Study the drawing (mm; zero at the part's minimum x, y, z) and answer. Coordinates: 2 decimals unless noted, no trailing zeros. Loops run counter-clockwise (first coordinate to the right, second up) from the corner with the lowest first, then second, coordinate; pieces in that order, holes last. Notation, with made-up numbers: (27.5, 41.25) - (38.5, 41.25) arc R17 cw to (38.5, 53.25) - close; hole circle Ø1 at (59, 28). An arc over 180 degrees is marked (long way). Write each question's results on one line, items separated by ' | '. Start each with the question number.
(1) Find section B-B on x = 28. Determine the outline of the cut face in (y, z).
(2) Find section C-C on z = 3.15. Determine the outline of the cut face in (x, y), then the cut area to 3 significant figures.
(3) Given pin 1 Ø1.5 at (x, z) = (66.5, 3) entering from +Y; pin 2 Ø5 at (x, y) = (95.165, 2.79) entering from +Z; pin 3 Ø2 at (y, z) = (18.5, 3.5) entering from -X, each flat-ended and moving along its own axis, determine where each tip first touches the part or whether it passes through.
(4) Consider line 1 (Y direction, x = 59.5, z = 2.3); line 2 (X direction, y = 3, z = 2.9). Determine where each line is inside the solid, lowest interval first. Write a range as from..to.
(5) Find section A-A on y = 49.5. Determine the outline of the cut face in (x, z).
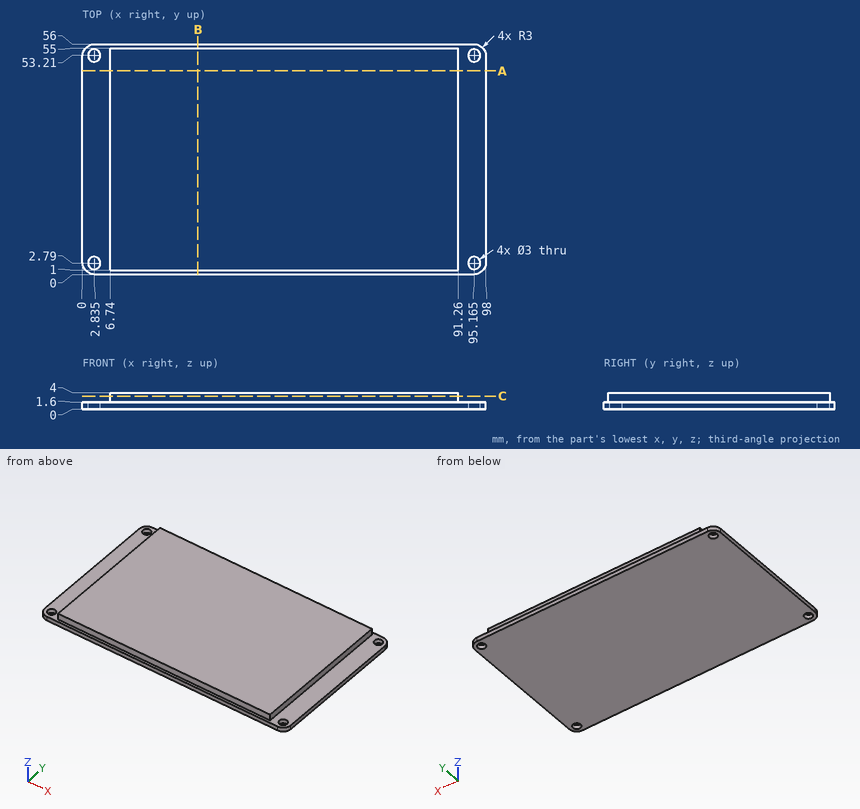
Values:
1) outline: (0, 0) - (56, 0) - (56, 1.6) - (55, 1.6) - (55, 4) - (1, 4) - (1, 1.6) - (0, 1.6) - close
2) outline: (6.74, 1) - (91.26, 1) - (91.26, 55) - (6.74, 55) - close | area: 4,560 mm²
3) pin 1: stops at y = 55 | pin 2: stops at z = 1.6 | pin 3: stops at x = 6.74
4) line 1: y = 1..55 | line 2: x = 6.74..91.26
5) outline: (0, 0) - (98, 0) - (98, 1.6) - (91.26, 1.6) - (91.26, 4) - (6.74, 4) - (6.74, 1.6) - (0, 1.6) - close
